For this review, use the dimensioned drawing (mm, ordinates from the lowest corner) and the shaded views. Coordinates: 2 decimals unless noted, no trailing zeros. Write each loop counter-clockwise with the first axis right and the second up, starting at its lowest first coordinate (ties: lowest second). Pieces come first, ordered by that corner, then holes. Notation, with made-up numbers: (22, 35) - (62, 35) arc R27 cw to (62, 62) - close; hole circle Ø3 at (0.5, 35). An arc over 180 degrees is marked (long way). One line per item, written item: value.
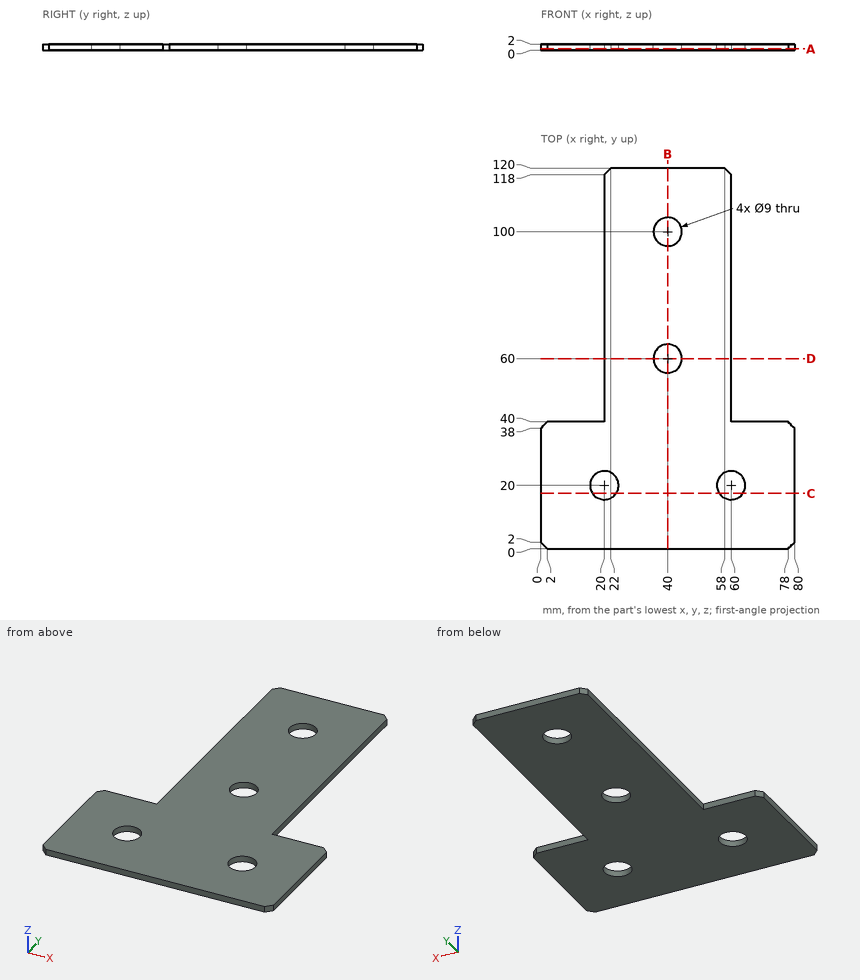
1. Consider section D-D, the plane y = 60. Write out the cut boundary in (x, z).
Answer block:
outline: (20, 0) - (35.5, 0) - (35.5, 2) - (20, 2) - close; (44.5, 0) - (60, 0) - (60, 2) - (44.5, 2) - close
2. Consider section A-A, the plane z = 0.5. Write out the cut boundary in (x, y), then the cut area to 3 significant figures.
Answer block:
outline: (0, 2) - (2, 0) - (78, 0) - (80, 2) - (80, 38) - (78, 40) - (60, 40) - (60, 118) - (58, 120) - (22, 120) - (20, 118) - (20, 40) - (2, 40) - (0, 38) - close; hole circle Ø9 at (20, 20); hole circle Ø9 at (40, 60); hole circle Ø9 at (40, 100); hole circle Ø9 at (60, 20)
area: 6,130 mm^2
3. Insertion check: pin 1 Ø8 at (x, y) = (20, 20) entering from +Z; pin 2 Ø1 at (y, z) = (102.5, 1) entering from -X; pin 3 Ø1 at (x, z) = (10, 0.5) entering from +Y. Each pin has a flat end and moves straight along its axis. Give the tip position at first contact, or say it passes through.
Answer block:
pin 1: passes through
pin 2: stops at x = 20
pin 3: stops at y = 40
4. Consider section B-B, the plane x = 40. Write out the cut boundary in (y, z).
Answer block:
outline: (0, 0) - (55.5, 0) - (55.5, 2) - (0, 2) - close; (64.5, 0) - (95.5, 0) - (95.5, 2) - (64.5, 2) - close; (104.5, 0) - (120, 0) - (120, 2) - (104.5, 2) - close
5. Consider section C-C, the plane y = 17.5. Write out the cut boundary in (x, z).
Answer block:
outline: (0, 0) - (16.26, 0) - (16.26, 2) - (0, 2) - close; (23.74, 0) - (56.26, 0) - (56.26, 2) - (23.74, 2) - close; (63.74, 0) - (80, 0) - (80, 2) - (63.74, 2) - close
6. Wall thickness on line 1 along Y through (x, z) = (40, 1.4); line 2 along X through (y, z) = (20, 1.4); line 3 along Y through (x, z) = (60.5, 0.5): over which ranges is each line inside the solid? List them lowest first.
Answer block:
line 1: y = 0 to 55.5, 64.5 to 95.5, 104.5 to 120
line 2: x = 0 to 15.5, 24.5 to 55.5, 64.5 to 80
line 3: y = 0 to 15.53, 24.47 to 40
